from build123d import *

# Parameters (mm, degrees)
F0_W     = 95
F0_H     = 32.5
F1_DEPTH = 12
F3_DEPTH = 10
F4_SIZE2 = 10
F4_SIZE  = 5


with BuildPart() as f1:
    # F0 (on Top) → F1 (new body)
    with BuildSketch(Plane.XY):
        with Locations((40.5, 9.25)):
            Rectangle(F0_W, F0_H)
    extrude(amount=F1_DEPTH)

    # F2 (on face) → F3 (cut)
    with BuildSketch(Plane.XY.offset(12)):
        Polygon((0, 18.5), (0, 0), (4.9286105492, 0), (81, 0), (81, 18.5), align=None)
    extrude(amount=-F3_DEPTH, mode=Mode.SUBTRACT)

    # F4
    f4_edges = [f1.edges().sort_by_distance(p)[0] for p in [
        (40.5, 25.5, 12),
        (88, 9.25, 12),
        (40.5, -7, 12),
        (-7, 9.25, 12),
    ]]
    f4_side = f1.faces().sort_by_distance((40.5, 24.495946, 12))[0]
    chamfer(f4_edges, length=F4_SIZE, length2=F4_SIZE2, reference=f4_side)


solid = f1.part
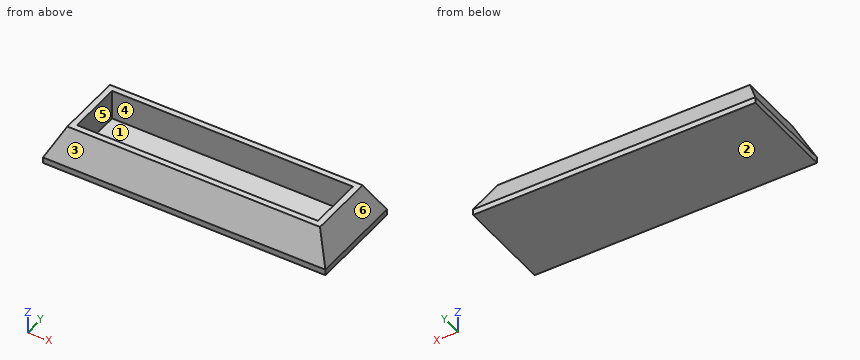
Work out the finished part from the listing and answer in its coordinate system (mm). Face numbers are marked on the shaded views. A direction names the side the tool comes from. Give positions to 0.01 mm unless a question says otherwise; leave off trailing zeros. Loops run counter-clockwise (first coordinate to the right, second up) from the corner with the lowest first, then second, coordinate; pieces in that order, holes last. Notation, with made-up numbers: (82.5, 51.25) - (123.5, 51.25) arc R8 ccw to (123.5, 60.25) - close; hole circle Ø6 at (44.5, 59.5). An arc over 180 degrees is marked (long way). Answer in a Markdown table with one row per item. Add a question column.
Q1. The part is cut by section D-D (z = 3.25). Determine the outline of the cut face in (x, y) (3 decimals), and give its area (3 significant figures).
Q2. The part is cut by section A-A (z = 9). Determine the outline of the cut face in (x, y), and give its area (4 significant figures).
Q3. Consider line 1 along X through (y, z) = (15, 11.5); line 2 along Y through (x, z) = (16, 5.75) (3 decimals); line 3 along X through (y, z) = (1.5, 5.75) (3 decimals). Determine where each line is inside the solid, lowest interval first.
Q4. A tool of negligible diameter and unlimited length cuts with its end or side. For the marked faces 1 and 2, from which of +Z, -Z, +X, -X, +Y, -Y can it reach the whole face along a straight path? Write none if from no direction.
Q5. The part is cut by section B-B (y = 12). Determine the outline of the cut face in (x, z).
Q6. Determine the mould class of the marked faces 3, 4, 5 and 6 for opening direction Y: released by +Y, released by -Y, zero draft, split by the parting line, or undercut.
Q7. The part is cut by section C-C (x = 71). Determine the outline of the cut face in (y, z).
Q8. Each of these flat-tipped pins is pushed along its axis until it touches: P1, Ø1.5, axis at y = 19, z = 3.5, coming from the +X side (3 decimals); P2, Ø6, axis at x = 77, y = 4, coming from the +Z side; P3, Ø3, axis at y = 7.5, z = 4.5, coming from the +X side. Where does it stop, or does it pass through?
Solution:
| question | item | result |
|---|---|---|
| 1 | outline | (-6.375, -6.375) - (87.375, -6.375) - (87.375, 24.875) - (-6.375, 24.875) - close; hole (0, 0) - (81, 0) - (81, 18.5) - (0, 18.5) - close |
| 1 | area | 1,430 mm² |
| 2 | outline | (-3.5, -3.5) - (84.5, -3.5) - (84.5, 22) - (-3.5, 22) - close; hole (0, 0) - (81, 0) - (81, 18.5) - (0, 18.5) - close |
| 2 | area | 745.5 mm² |
| 3 | line 1 | x = -2.25 to 0, 81 to 83.25 |
| 3 | line 2 | y = -5.125 to 0, 18.5 to 23.625 |
| 3 | line 3 | x = -5.125 to 0, 81 to 86.125 |
| 4 | face 1 | +Z |
| 4 | face 2 | -Z, +X, -X, +Y, -Y |
| 5 | outline | (-7, 0) - (88, 0) - (88, 2) - (83, 12) - (81, 12) - (81, 2) - (0, 2) - (0, 12) - (-2, 12) - (-7, 2) - close |
| 6 | face 3 | released by -Y |
| 6 | face 4 | undercut |
| 6 | face 5 | undercut |
| 6 | face 6 | zero draft |
| 7 | outline | (-7, 0) - (25.5, 0) - (25.5, 2) - (20.5, 12) - (18.5, 12) - (18.5, 2) - (0, 2) - (0, 12) - (-2, 12) - (-7, 2) - close |
| 8 | P1 | stops at x = 87.625 |
| 8 | P2 | stops at z = 2 |
| 8 | P3 | stops at x = 87.5 |
